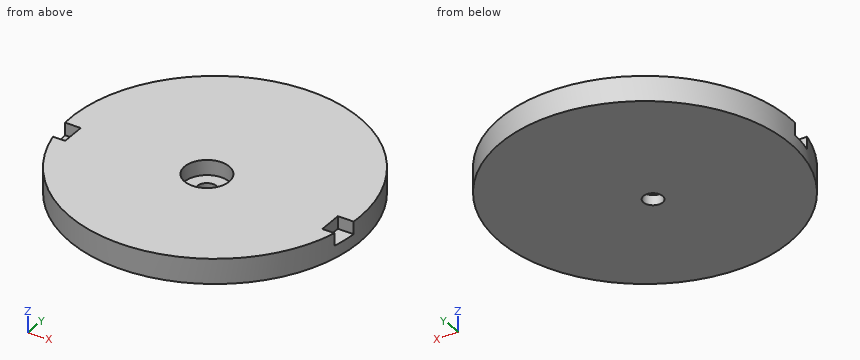
from build123d import *

# Parameters (mm, degrees)
SKETCH1_R           = 73.406
BOSS_EXTRUDE1_DEPTH = 12.7
CUT_EXTRUDE1_DEPTH  = 6.35
SKETCH3_R           = 11.303
CUT_EXTRUDE2_DEPTH  = 7.62
SKETCH4_R           = 4.8641
CUT_EXTRUDE3_DEPTH  = 105.585714474


with BuildPart() as part:
    # Sketch1 → Boss-Extrude1 (new body)
    with BuildSketch(Plane.XY):
        Circle(SKETCH1_R)
    extrude(amount=-BOSS_EXTRUDE1_DEPTH)

    # Sketch2 → Cut-Extrude1 (cut)
    with BuildSketch(Plane.XY):
        Polygon((-71.466139815, -4.4958), (-71.466139815, -16.764), (-65.268539815, -16.764), (-65.268539815, -4.4958), (-67.31, -4.4958), align=None)
        with BuildLine():
            ThreePointArc((-73.2681965, -4.4958), (-72.626676985, -10.668018845), (-71.466139815, -16.764))
            Line((-71.466139815, -16.764), (-71.466139815, -4.4958))
            Line((-71.466139815, -4.4958), (-73.2681965, -4.4958))
        make_face()
        Polygon((71.466139815, -16.764), (71.466139815, -4.4958), (67.31, -4.4958), (65.268539815, -4.4958), (65.268539815, -16.764), align=None)
        with BuildLine():
            Line((73.2681965, -4.4958), (71.466139815, -4.4958))
            Line((71.466139815, -4.4958), (71.466139815, -16.764))
            ThreePointArc((71.466139815, -16.764), (72.626676985, -10.668018845), (73.2681965, -4.4958))
        make_face()
    extrude(amount=-CUT_EXTRUDE1_DEPTH, mode=Mode.SUBTRACT)

    # Sketch3 → Cut-Extrude2 (cut)
    with BuildSketch(Plane.XY):
        with Locations((0, -6.35)):
            Circle(SKETCH3_R)
    extrude(amount=-CUT_EXTRUDE2_DEPTH, mode=Mode.SUBTRACT)

    # Sketch4 → Cut-Extrude3 (cut, through all)
    with BuildSketch(Plane.XY):
        with Locations((0, -6.35)):
            Circle(SKETCH4_R)
    extrude(amount=-CUT_EXTRUDE3_DEPTH, mode=Mode.SUBTRACT)


solid = part.part
Input: part model. Units: mm. Frame: model coordinates. Give positions to 0.01 mm unless a question says otherwise; leave off trailing zeros. Write each loop counter-clockwise with the first axis right and the second up, starting at its lowest first coordinate (ties: lowest second). Pieces come first, ordered by that corner, then holes.
Q1. First-contact query: P1, Ø3, axis at x = -69, z = -2.5, coming from the +Y side; P2, Ø7, axis at x = -71, z = -3.5, coming from the -Y side; P3, Ø4, axis at y = 52, z = -10, coming from the -X side. Flat tips, straight axial feed; report the tip coordinate or a pass-through.
Q2. Section C-C, the plane z = -9.75. Output: boundary loops of the cut face in (x, y), plus the area to 3 significant figures.
Q3. Section A-A, the plane x = 0. Output: boundary loops of the cut face in (y, z).
Q4. Material intervals for probe 1 along Y at (x, z) = (0, -4.75); probe 2 along Z at (x, y) = (-3.5, -14.5); probe 3 along X at (y, z) = (0.5, -7), sorted ascending.
Q5. Section B-B, the plane y = -6.35. Output: boundary loops of the cut face in (x, z).
Q6. Section D-D, the plane y = 29. Output: boundary loops of the cut face in (x, z).
Filled in:
1. P1: stops at y = 28.85
1. P2: stops at y = -28.85
1. P3: stops at x = -53.74
2. outline: circle Ø146.81 at (0, 0); hole circle Ø9.73 at (0, -6.35)
2. area: 16,900 mm2
3. outline: (-73.41, -12.7) - (-11.21, -12.7) - (-11.21, -7.62) - (-17.65, -7.62) - (-17.65, 0) - (-73.41, 0) - close; (-1.49, -12.7) - (73.41, -12.7) - (73.41, 0) - (4.95, 0) - (4.95, -7.62) - (-1.49, -7.62) - close
4. probe 1: y = -73.41 to -17.65, 4.95 to 73.41
4. probe 2: z = -12.7 to -7.62
4. probe 3: x = -73.4 to -8.99, 8.99 to 73.4
5. outline: (-73.13, -12.7) - (-4.86, -12.7) - (-4.86, -7.62) - (-11.3, -7.62) - (-11.3, 0) - (-65.27, 0) - (-65.27, -6.35) - (-73.13, -6.35) - close; (4.86, -12.7) - (73.13, -12.7) - (73.13, -6.35) - (65.27, -6.35) - (65.27, 0) - (11.3, 0) - (11.3, -7.62) - (4.86, -7.62) - close
6. outline: (-67.43, -12.7) - (67.43, -12.7) - (67.43, 0) - (-67.43, 0) - close
